Input: part model. Units: mm. Frame: model coordinates. A direction names the side the tool comes from. Give positions to 0.01 mm unless a question says otherwise; leave off trailing zeros. Loops run counter-clockwise (first coordinate to the right, second up) from the corner with the lowest first, then second, coordinate; pieces in that order, holes last. Notation, with made-up numbers: M 71.25,89.25 L 120.25,89.25 A25 ccw 120.25,108.25 Z; hole C 48.25,22 d2. An arc over 180 degrees is marked long. Use a Markdown table: item, result. Add a question column.
from build123d import *

# Parameters (mm, degrees)
F0_W      = 50.8
F0_H      = 16.9333164
F1_DEPTH  = 50.8
F2_R      = 25.39999
F4_DEPTH  = 119.50414
F5_R      = 3.175
F6_DEPTH  = 61.82298
F7_R      = 3.175
F8_DEPTH  = 63.51287
F9_W      = 38.1
F9_H      = 12.7
F10_DEPTH = 114.99064


# Not quite as in the source:
# - a fillet or chamfer is up to 0.001 mm smaller than in the source, because OpenCascade refuses the exact size


with BuildPart() as f1:
    # F0 (on Top) → F1 (new body)
    with BuildSketch(Plane.XY):
        Polygon((-50.8, 0), (0, 0), (0, 29.633350436), (0, 46.566666836), (0, 76.2), (-50.8, 76.2), (-50.8, 50.8), (-25.4, 50.8), (-25.4, 25.4), (-50.8, 25.4), align=None)
        with Locations((25.4, 38.100008636)):
            Rectangle(F0_W, F0_H)
    extrude(amount=F1_DEPTH)

    # F2 (radius 25.4 in the source; OpenCascade refuses exactly that, so slightly less here)
    f2_edges = [f1.edges().sort_by_distance(p)[0] for p in [
        (50.8, 38.100009, 50.8),
        (50.8, 38.100009, 0),
    ]]
    fillet(f2_edges, radius=F2_R)

    # F3 (on face) → F4 (cut)
    with BuildSketch(Plane.XZ):
        Polygon((-50.8, 50.8), (-50.8, 38.1), (0, 50.8), align=None)
        Polygon((0, 0), (-50.8, 12.7), (-50.8, 0), align=None)
    extrude(amount=-F4_DEPTH, mode=Mode.SUBTRACT)

    # F5 (on face) → F6 (cut)
    with BuildSketch(Plane.XZ.offset(-29.633350436)):
        with Locations((25.4, 25.4)):
            Circle(F5_R)
    extrude(amount=-F6_DEPTH, mode=Mode.SUBTRACT)

    # F7 (on face) → F8 (cut)
    with BuildSketch(Plane.XY):
        with Locations((-38.1, 12.7)):
            Circle(F7_R)
        with Locations((-38.1, 63.5)):
            Circle(F7_R)
    extrude(amount=F8_DEPTH, mode=Mode.SUBTRACT)

    # F9 (on face) → F10 (cut)
    with BuildSketch(Plane.XZ):
        with Locations((-31.75, 25.4)):
            Rectangle(F9_W, F9_H)
    extrude(amount=-F10_DEPTH, mode=Mode.SUBTRACT)


solid = f1.part
1) Section query A-A, the plane x = -20. Return the cut outline in (y, z), and give its area (3 significant figures).
2) Pull-direction query (X, two-part tool) for faces 1 (the flat face through (13, 38, 0)), 2 (the flat face through (-19.4, 37.57, 4.85)), 3 (the cylindrical face through (28.43, 37.98, 26.35)); classes: pulls with the +X half, pulls with the -X half, needs draft (parallel to the pull), parting line crosses it, or undercut.
3) Section query C-C, the plane z = 11. Return the cut outline in (x, y) (3 decimals), and give its area (3 significant figures).
4) Reachability of faces 4 (the flat face through (0, 15, 25)), 5 (the flat face through (-38, 25.4, 37)), 6 (the flat face through (-24, 38, 19.05)) from +Z, -Z, +X, -X, +Y, -Y: full face, straight path, thin tool, end or side. Return the list, or none.
5) Section query B-B, the plane y = 12.7. Return the cut outline in (x, z) (3 decimals), and give its area (3 significant figures).
6) Contact query for flat-ended pins moving along their axis: P1, Ø1.5, axis at y = 16.5, z = 13.5, coming from the +X side; P2, Ø4, axis at x = -26.5, y = 9.5, coming from the +Z side (3 decimals); P3, Ø1, axis at x = 25.5, z = 41.5, coming from the -Y side. Output: stop coordinate, or through.
7) Ray query, line 1 (Y direction, x = -38.1, z = 13.5) (3 decimals); line 2 (Z direction, x = 25.4, y = 36.5) (3 decimals); line 3 (Y direction, x = -33, z = 33). Return the intervals inside material, ascending. Write a range as [from, to].
Entries:
| question | item | result |
|---|---|---|
| 1 | outline | M 0,5 L 76.2,5 L 76.2,19.05 L 0,19.05 Z; M 0,31.75 L 76.2,31.75 L 76.2,45.8 L 0,45.8 Z |
| 1 | area | 2,140 mm² |
| 2 | face 1 | needs draft |
| 2 | face 2 | pulls with the -X half |
| 2 | face 3 | undercut |
| 3 | outline | M -44,0 L 0,0 L 0,29.633 L 46.324,29.633 L 46.324,46.567 L 0,46.567 L 0,76.2 L -44,76.2 L -44,50.8 L -25.4,50.8 L -25.4,25.4 L -44,25.4 Z; hole C -38.1,12.7 d6.35; hole C -38.1,63.5 d6.35 |
| 3 | area | 3,600 mm² |
| 4 | face 4 | +Z, -Z, +X, -Y |
| 4 | face 5 | +Z, -Z, -X |
| 4 | face 6 | -X, +Y, -Y |
| 5 | outline | M -50.8,12.7 L -41.275,10.319 L -41.275,19.05 L -50.8,19.05 Z; M -50.8,31.75 L -41.275,31.75 L -41.275,40.481 L -50.8,38.1 Z; M -34.925,8.731 L 0,0 L 0,50.8 L -34.925,42.069 L -34.925,31.75 L -12.7,31.75 L -12.7,19.05 L -34.925,19.05 Z |
| 5 | area | 1,330 mm² |
| 6 | P1 | stops at x = 0 |
| 6 | P2 | stops at z = 44.675 |
| 6 | P3 | stops at y = 29.63 |
| 7 | line 1 | y = [0, 9.525], [15.875, 25.4], [50.8, 60.325], [66.675, 76.2] |
| 7 | line 2 | z = [0, 22.225], [28.575, 50.8] |
| 7 | line 3 | y = [0, 25.4], [50.8, 76.2] |
